Verification items for the finished model (mm, model axes). Round coordinates to 2 decimals unless told otherwise and drop trailing zeros. Write each loop counter-clockwise with the first axis right and the second up, starting at its lowest first coordinate (ties: lowest second). Pieces come first, ordered by that corner, then holes. Notation, with made-up numbers: (-5, 28) -> (37, 28) arc R27 cw to (37, 44) -> close; hole circle Ø8 at (11, 22). An arc over 180 degrees is marked (long way). Answer as a JSON object with one key per item and string values. Group by question number.
(1) Scan lines: L1, parallel to Y at x = 2.3, z = 0; L2, parallel to Z at x = 1.85, y = 130; L3, parallel to Z at x = 0.95, y = -128. Record each from-to range of solid material in increasing order. Write a range as from..to.
(2) Sectioned sample at B-B on y = -125. Record the cut outline in (x, z).
(3) Draft check along Z on faces 1 (the face through (1.52, 132.53, -1.61)), 2 (the face through (3, 2, 0)). Enter one of: released by +Z, released by -Z, zero draft, split by the parting line, or undercut.
(4) Gauge pin test, flat ends, axial feed: pin 1 Ø1.5 at (x, z) = (1.5, 4) entering from -Y; pin 2 Ø5.5 at (y, z) = (130, 0) entering from +X. Record the tip position at first contact, or that the pin passes through.
(5) Sectioned sample at A-A on y = 130. Record the cut outline in (x, z), and give its area (3 significant figures).
```python
from build123d import *

# Parameters (mm, degrees)
SKETCH1_W           = 40
SKETCH1_H           = 300
BOSS_EXTRUDE1_DEPTH = 3
SKETCH2_R           = 3
CUT_EXTRUDE1_DEPTH  = 3
SKETCH3_W           = 3
SKETCH3_H           = 27.5
CUT_EXTRUDE2_DEPTH  = 3


with BuildPart() as part:
    # Sketch1 → Boss-Extrude1 (new body)
    with BuildSketch(Plane(origin=(0, 0, 0), x_dir=(0, 0, -1), z_dir=(1, 0, 0))):
        Rectangle(SKETCH1_W, SKETCH1_H)
    extrude(amount=BOSS_EXTRUDE1_DEPTH)

    # Sketch2 → Cut-Extrude1 (cut)
    with BuildSketch(Plane(origin=(3, 0, 0), x_dir=(0, 0, -1), z_dir=(1, 0, 0))):
        with Locations((0, 130)):
            Circle(SKETCH2_R)
    extrude(amount=-CUT_EXTRUDE1_DEPTH, mode=Mode.SUBTRACT)

    # Sketch3 → Cut-Extrude2 (cut)
    with BuildSketch(Plane(origin=(3, 0, 0), x_dir=(0, 0, -1), z_dir=(1, 0, 0))):
        with Locations((-3.5, -136.25)):
            Rectangle(SKETCH3_W, SKETCH3_H)
    extrude(amount=-CUT_EXTRUDE2_DEPTH, mode=Mode.SUBTRACT)


solid = part.part
```
Computed values:
{
 "1": {"L1": "-150..127, 133..150", "L2": "-20..-3, 3..20", "L3": "-20..2, 5..20"},
 "2": {"outline": "(0, -20) -> (3, -20) -> (3, 2) -> (0, 2) -> close; (0, 5) -> (3, 5) -> (3, 20) -> (0, 20) -> close"},
 "3": {"face 1": "undercut", "face 2": "zero draft"},
 "4": {"pin 1": "y = -122.5", "pin 2": "through"},
 "5": {"outline": "(0, -20) -> (3, -20) -> (3, -3) -> (0, -3) -> close; (0, 3) -> (3, 3) -> (3, 20) -> (0, 20) -> close", "area": "102 mm2"}
}
